```python
from build123d import *

# Parameters (mm, degrees)
BOSS_EXTRUDE1_DEPTH      = 14.605
BOSS_EXTRUDE1_DEPTH_BACK = 3.175
SKETCH1_R                = 4.7625
CUT_EXTRUDE1_DEPTH       = 20.32
SKETCH4_R                = 2.2225
CUT_EXTRUDE2_DEPTH       = 20.32
SKETCH5_R                = 4.445
BOSS_EXTRUDE2_DEPTH      = 17.78
SKETCH6_R                = 1.397
CUT_EXTRUDE3_DEPTH       = 17.78


with BuildPart() as part:
    # Sketch2 → Boss-Extrude1 (new body, two sides)
    with BuildSketch(Plane(origin=(0, 0, 0), x_dir=(1, 0, 0), z_dir=(0, 1, 0))) as boss_extrude1_sk:
        with BuildLine():
            ThreePointArc((-6.35, 7.099515829), (-7.099515829, -6.35), (6.35, -7.099515829))
            ThreePointArc((6.35, -7.099515829), (42.007194804, 3.857031119), (77.664389608, -7.099515829))
            ThreePointArc((77.664389608, -7.099515829), (91.113905436, -6.35), (90.364389608, 7.099515829))
            ThreePointArc((90.364389608, 7.099515829), (42.007194804, 22.745971747), (-6.35, 7.099515829))
        make_face()
    extrude(amount=BOSS_EXTRUDE1_DEPTH)
    extrude(boss_extrude1_sk.sketch, amount=-BOSS_EXTRUDE1_DEPTH_BACK)

    # Sketch1 → Cut-Extrude1 (cut)
    with BuildSketch(Plane(origin=(0, 0, 0), x_dir=(1, 0, 0), z_dir=(0, 1, 0))):
        Circle(SKETCH1_R)
        with Locations((13.367402776, 6.886065441)):
            Circle(SKETCH1_R)
        with Locations((70.646986832, 6.886065441)):
            Circle(SKETCH1_R)
        with Locations((84.014389608, 0)):
            Circle(SKETCH1_R)
    extrude(amount=CUT_EXTRUDE1_DEPTH, mode=Mode.SUBTRACT)

    # Sketch4 → Cut-Extrude2 (cut)
    with BuildSketch(Plane(origin=(0, 0, 0), x_dir=(1, 0, 0), z_dir=(0, 1, 0))):
        with Locations((13.367402776, 6.886065441)):
            Circle(SKETCH4_R)
        Circle(SKETCH4_R)
        with Locations((70.646986832, 6.886065441)):
            Circle(SKETCH4_R)
        with Locations((84.014389608, 0)):
            Circle(SKETCH4_R)
    extrude(amount=-CUT_EXTRUDE2_DEPTH, mode=Mode.SUBTRACT)

    # Sketch5 → Boss-Extrude2 (add)
    with BuildSketch(Plane(origin=(0, 14.605, 0), x_dir=(1, 0, 0), z_dir=(0, 1, 0))):
        with Locations((-7.62, -6.35)):
            Circle(SKETCH5_R)
        with Locations((91.634389608, -6.35)):
            Circle(SKETCH5_R)
    extrude(amount=-BOSS_EXTRUDE2_DEPTH)

    # Sketch6 → Cut-Extrude3 (cut)
    with BuildSketch(Plane(origin=(0, 14.605, 0), x_dir=(1, 0, 0), z_dir=(0, 1, 0))):
        with Locations((42.007194804, 13.97)):
            Circle(SKETCH6_R)
        with Locations((-7.62, -6.35)):
            Circle(SKETCH6_R)
        with Locations((91.634389608, -6.35)):
            Circle(SKETCH6_R)
    extrude(amount=-CUT_EXTRUDE3_DEPTH, mode=Mode.SUBTRACT)


solid = part.part
```
Part model, mm, in its own coordinate system. A direction names the side the tool comes from. Give positions to 0.01 mm unless a question says otherwise; leave off trailing zeros. Loops run counter-clockwise (first coordinate to the right, second up) from the corner with the lowest first, then second, coordinate; pieces in that order, holes last. Notation, with made-up numbers: M 56.25,28 L 66.25,28 A18 ccw 66.25,51 Z; hole C 59.5,27.5 d10. An arc over 180 degrees is marked long. Return JSON: item names as keys, results as strings.
1) Saw through at C-C, the plane x = 0. List the corners of the cut face in (y, z) (1 decimal).
Calculated:
{"outline": "M -3.2,-11.3 L 14.6,-11.3 L 14.6,-4.8 L 0,-4.8 L 0,-2.2 L -3.2,-2.2 Z; M -3.2,2.2 L 0,2.2 L 0,4.8 L 14.6,4.8 L 14.6,9.5 L -3.2,9.5 Z"}
2) Saw through at A-A, the plane z = -13.97. List the corners of the cut face in (x, y) (3 decimals).
Calculated:
{"outline": "M 4.968,-3.175 L 40.61,-3.175 L 40.61,14.605 L 4.968,14.605 Z; M 43.404,-3.175 L 79.046,-3.175 L 79.046,14.605 L 43.404,14.605 Z"}
3) Saw through at B-B, the plane y = 3.25. Count the separate pieces of the cut face and the enclosed holes in it, then the cut area to 3 significant figures.
Calculated:
{"separate pieces": "1", "enclosed holes": "7", "area": "1,750 mm2"}
4) Pull direction X, two halves, no side cores. Call faces 1 (the face through (41, 14.605, -6)), 2 (the face through (-9.07, 5.84, -2.91)), 3 (the face through (41.477, 5.839, -3.855)), 4 (the face through (42.73, 5.839, -22.743)): released by +X, released by -X, zero draft, split by the parting line, or undercut.
Calculated:
{"face 1": "zero draft", "face 2": "released by -X", "face 3": "undercut", "face 4": "split by the parting line"}
5) Saw through at D-D, the plane z = 0. List the corners of the cut face in (x, y) (1 decimal).
Calculated:
{"outline": "M -9.5,-3.2 L -2.2,-3.2 L -2.2,0 L -4.8,0 L -4.8,14.6 L -9.5,14.6 Z; M 2.2,-3.2 L 20.2,-3.2 L 20.2,14.6 L 4.8,14.6 L 4.8,0 L 2.2,0 Z; M 63.8,-3.2 L 81.8,-3.2 L 81.8,0 L 79.3,0 L 79.3,14.6 L 63.8,14.6 Z; M 86.2,-3.2 L 93.5,-3.2 L 93.5,14.6 L 88.8,14.6 L 88.8,0 L 86.2,0 Z"}
6) 3-axis set-ups, long thin cutter, end or side, ignore diameter. For faces 5 (the face through (15.42, -1.57, -6.03)), 6 (the face through (65.89, 7.2, -7.1)): which of +Z, -Z, +X, -X, +Y, -Y reach the whole face in a straight line?
Calculated:
{"face 5": "+Y, -Y", "face 6": "+Y"}
7) Flat gauge pins, fed straight in: pin 1 Ø3 at (x, z) = (91.63, 6.35) entering from +Y (3 decimals); pin 2 Ø5.5 at (x, z) = (70.65, -6.89) entering from +Y; pin 3 Ø10 at (y, z) = (8, -0.5) entering from -X; pin 4 Ø1 at (x, y) = (-1, 2) entering from +Z. Where does each tip first touch, or does it go through?
Calculated:
{"pin 1": "stops at y = 14.605", "pin 2": "stops at y = 0", "pin 3": "stops at x = -11.66", "pin 4": "stops at z = 9.51"}
8) Drill centre lines: line 1 (X direction, y = 5, z = 6.35) (3 decimals); line 2 (X direction, y = 5, z = 6); line 3 (X direction, y = 6, z = -6). Where is each one in solid material? Low to high.
Calculated:
{"line 1": "x = -12.065 to -9.017, -6.223 to 7.48, 76.534 to 90.237, 93.031 to 96.079", "line 2": "x = -12.05 to -8.97, -6.27 to 8.03, 75.99 to 90.28, 92.99 to 96.07", "line 3": "x = -7.4 to 8.69, 18.05 to 65.97, 75.33 to 91.41"}
